Verification items for the finished model (mm, model axes). Coordinates: 2 decimals unless noted, no trailing zeros. Write each loop counter-clockwise with the first axis right and the second up, starting at its lowest first coordinate (ties: lowest second). Pieces come first, ordered by that corner, then holes. Notation, with made-up numbers: (63.25, 73) - (117.25, 73) arc R24 cw to (117.25, 87) - close; hole circle Ø2 at (56, -37). An arc over 180 degrees is marked (long way). Answer as CSV lines item,"result". Start each with the question number.
```python
from build123d import *

# Parameters (mm, degrees)
DODANIE_WYCI_GNI_CIE1_OUTLINE_R = 3.000000079
DODANIE_WYCI_GNI_CIE1_DEPTH     = 5
SZKIC2_W                        = 1.618528634
SZKIC2_H                        = 4.134107934
SZKIC2_H_2                      = 3.371537851
SZKIC2_W_2                      = 0.651830256
SZKIC2_H_3                      = 2.48709631
SZKIC2_H_4                      = 2.564588173
WYTNIJ_WYCI_GNI_CIE3_DEPTH      = 194.428536027


# Read off the part's stored shape, not the designer's step: Dodanie-wyciągnięcie1
with BuildPart() as part:
    # Dodanie-wyciągnięcie1 outline → Dodanie-wyciągnięcie1 (new body)
    with BuildSketch(Plane.XY):
        with BuildLine():
            Line((187.7624, 5.522620658), (0, 4.635188213))
            ThreePointArc((0, 4.635188213), (-4.635188213, 0), (0, -4.635188213))
            Line((0, -4.635188213), (187.7624, -5.522620658))
            ThreePointArc((187.7624, -5.522620658), (193.285020658, 0), (187.7624, 5.522620658))
        make_face()
        Circle(DODANIE_WYCI_GNI_CIE1_OUTLINE_R, mode=Mode.SUBTRACT)
        with Locations((187.7624, 0)):
            Circle(DODANIE_WYCI_GNI_CIE1_OUTLINE_R, mode=Mode.SUBTRACT)
    extrude(amount=DODANIE_WYCI_GNI_CIE1_DEPTH)

    # Szkic2 → Wytnij-wyciągnięcie3 (cut, through all)
    with BuildSketch(Plane.XY):
        with Locations((193.638606269, 2.067053967)):
            Rectangle(SZKIC2_W, SZKIC2_H)
        with Locations((193.638606269, -1.685768926)):
            Rectangle(SZKIC2_W, SZKIC2_H_2)
        with Locations((-4.682734605, 1.243548155)):
            Rectangle(SZKIC2_W_2, SZKIC2_H_3)
        with Locations((-4.682734605, -1.282294087)):
            Rectangle(SZKIC2_W_2, SZKIC2_H_4)
    extrude(amount=WYTNIJ_WYCI_GNI_CIE3_DEPTH, mode=Mode.SUBTRACT)


solid = part.part
```
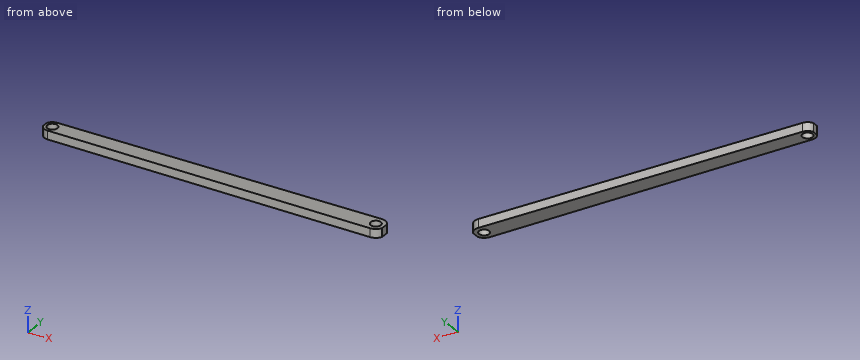
1. Cross-section at B-B (z = 2.1). Record the cut outline in (x, y), and give its area (3 significant figures).
2. Cross-section at D-D (x = 132). Record the cut outline in (y, z), and give its area (3 significant figures).
3. Depth check by flat-ended pin: P1, Ø1.5, axis at y = -3.5, z = 3.5, coming from the +X side. Enter the tip coordinate at first touch or a pass-through.
4. Cross-section at A-A (y = 0). Record the cut outline in (x, z).
5. Cross-section at C-C (x = 158.5). Record the cut outline in (y, z).
6. Scan lines: line 1 along X through (y, z) = (0.25, 3.05); line 2 along X through (y, z) = (0.5, 0.8); line 3 along Y through (x, z) = (0, 2.55). Record each from-to range of solid material in increasing order. Write a range as from..to.
Completed:
1,outline,"(-4.36, -1.58) arc R4.64 ccw to (0, -4.64) - (187.76, -5.52) arc R5.52 ccw to (192.83, -2.2) - (192.83, 2.2) arc R5.52 ccw to (187.76, 5.52) - (0, 4.64) arc R4.64 ccw to (-4.36, 1.58) - close; hole circle Ø6 at (0, 0); hole circle Ø6 at (187.76, 0)"
1,area,"1,930 mm2"
2,outline,"(-5.26, 0) - (5.26, 0) - (5.26, 5) - (-5.26, 5) - close"
2,area,"52.6 mm2"
3,P1,"stops at x = 192.55"
4,outline,"(-4.36, 0) - (-3, 0) - (-3, 5) - (-4.36, 5) - close; (3, 0) - (184.76, 0) - (184.76, 5) - (3, 5) - close; (190.76, 0) - (192.83, 0) - (192.83, 5) - (190.76, 5) - close"
5,outline,"(-5.38, 0) - (5.38, 0) - (5.38, 5) - (-5.38, 5) - close"
6,line 1,"x = -4.36..-2.99, 2.99..184.77, 190.75..192.83"
6,line 2,"x = -4.36..-2.96, 2.96..184.8, 190.72..192.83"
6,line 3,"y = -4.64..-3, 3..4.64"
